from build123d import *

# Parameters (mm, degrees)
SKETCH1_W           = 25
SKETCH1_H           = 50
SKETCH1_R           = 3.375
BOSS_EXTRUDE1_DEPTH = 3
SKETCH2_W           = 50
SKETCH2_H           = 3
BOSS_EXTRUDE2_DEPTH = 8
SKETCH3_W           = 8
SKETCH3_H           = 50
BOSS_EXTRUDE3_DEPTH = 42
SKETCH4_R           = 2.65
CUT_EXTRUDE1_DEPTH  = 3.3
SKETCH5_R           = 5.802370205
CUT_EXTRUDE2_DEPTH  = 9
FILLET2_R           = 1
SKETCH6_R           = 12.7
BOSS_EXTRUDE4_DEPTH = 2
FILLET4_R           = 1
SKETCH8_R           = 1.589780168
SKETCH8_R_2         = 1.777428262
CUT_EXTRUDE3_DEPTH  = 10
SKETCH9_W           = 8
SKETCH9_H           = 42
CUT_EXTRUDE4_DEPTH  = 68.79439129
SKETCH10_W          = 33.517939775
SKETCH10_H          = 6.212330843
CUT_EXTRUDE5_DEPTH  = 55


with BuildPart() as part:
    # Sketch1 → Boss-Extrude1 (new body)
    with BuildSketch(Plane(origin=(0, 0, 0), x_dir=(1, 0, 0), z_dir=(0, 1, 0))):
        with Locations((2.276951673, 11.384758364)):
            Rectangle(SKETCH1_W, SKETCH1_H)
        with Locations(Location((1.276951673, 11.384758364, 0), (0, 0, 270))):
            Circle(SKETCH1_R, mode=Mode.SUBTRACT)
    extrude(amount=BOSS_EXTRUDE1_DEPTH)

    # Sketch2 → Boss-Extrude2 (add)
    with BuildSketch(Plane.ZY.offset(10.223048327)):
        with Locations((-11.384758364, 1.5)):
            Rectangle(SKETCH2_W, SKETCH2_H)
    extrude(amount=BOSS_EXTRUDE2_DEPTH)

    # Sketch3 → Boss-Extrude3 (add)
    with BuildSketch(Plane.XZ):
        with Locations((-14.223048327, -11.384758364)):
            Rectangle(SKETCH3_W, SKETCH3_H)
    extrude(amount=BOSS_EXTRUDE3_DEPTH)

    # Sketch4 → Cut-Extrude1 (cut)
    with BuildSketch(Plane(origin=(0, 3, 0), x_dir=(1, 0, 0), z_dir=(0, 1, 0))):
        with Locations(Location((-14.223048327, 32.384758364, 0), (0, 0, 270))):
            Circle(SKETCH4_R)
        with Locations(Location((-14.223048327, -9.615241636, 0), (0, 0, 270))):
            Circle(SKETCH4_R)
    cut_extrude1 = extrude(amount=-CUT_EXTRUDE1_DEPTH, mode=Mode.SUBTRACT)

    # Mirror1: Cut-Extrude1 across plane
    add(cut_extrude1.mirror(Plane.ZX.offset(-19.5)), mode=Mode.SUBTRACT)

    # Sketch5 → Cut-Extrude2 (cut)
    with BuildSketch(Plane.ZY.offset(18.223048327)):
        with Locations((-11.836279124, -21)):
            Circle(SKETCH5_R)
    extrude(amount=-CUT_EXTRUDE2_DEPTH, mode=Mode.SUBTRACT)

    # Fillet2
    fillet2_edges = [part.edges().sort_by_distance(p)[0] for p in [
        (-10.223048327, -21, -17.638649329),
    ]]
    fillet(fillet2_edges, radius=FILLET2_R)

    # Mirror2: Cut-Extrude1 across plane
    add(cut_extrude1.mirror(Plane.ZY.offset(1.723048327)), mode=Mode.SUBTRACT)

    # Sketch6 → Boss-Extrude4 (add)
    with BuildSketch(Plane(origin=(0, 3, 0), x_dir=(1, 0, 0), z_dir=(0, 1, 0))):
        with BuildLine():
            Line((14.776951673, 5.567542535), (14.776951673, 17.201974193))
            ThreePointArc((14.776951673, 17.201974193), (-13.423048327, 11.384758364), (14.776951673, 5.567542535))
        make_face()
        with Locations(Location((1.276951673, 11.384758364, 0), (0, 0, 270))):
            Circle(SKETCH6_R, mode=Mode.SUBTRACT)
    extrude(amount=BOSS_EXTRUDE4_DEPTH)

    # Fillet4
    # the kernel refuses this fillet: 1 mm, written as the material it takes off along each edge
    with BuildSketch(Plane(origin=(14.776951673, 5, -3.067542535), x_dir=(0, -1, 0), z_dir=(0, 0, -1))) as fillet4_piece_1:
        with BuildLine():
            CenterArc((FILLET4_R, FILLET4_R), FILLET4_R, 180, 90)
            Line((0, FILLET4_R), (0, 0))
            Line((0, 0), (FILLET4_R, 0))
        make_face()
    extrude(amount=16.634431658, mode=Mode.SUBTRACT)

    # Sketch8 → Cut-Extrude3 (cut)
    with BuildSketch(Plane(origin=(0, 3, 0), x_dir=(1, 0, 0), z_dir=(0, 1, 0))):
        with Locations(Location((1.276951673, 19.884758364, 0), (0, 0, 270))):
            Circle(SKETCH8_R)
        with Locations(Location((1.276951673, 2.884758364, 0), (0, 0, 270))):
            Circle(SKETCH8_R_2)
    extrude(amount=-CUT_EXTRUDE3_DEPTH, mode=Mode.SUBTRACT)

    # Sketch9 → Cut-Extrude4 (cut, through all)
    with BuildSketch(Plane.XY.offset(13.615241636)):
        with Locations((-14.223048327, -21)):
            Rectangle(SKETCH9_W, SKETCH9_H)
    extrude(amount=-CUT_EXTRUDE4_DEPTH, mode=Mode.SUBTRACT)

    # Sketch10 → Cut-Extrude5 (cut)
    with BuildSketch(Plane.XY.offset(13.615241636)):
        with Locations((-1.464078439, 6.106165422)):
            Rectangle(SKETCH10_W, SKETCH10_H)
    extrude(amount=-CUT_EXTRUDE5_DEPTH, mode=Mode.SUBTRACT)


solid = part.part
Source: CAD feature listing. Evaluate the final solid. Frame: model axes, mm. Coordinates: 2 decimals unless noted, no trailing zeros. Loops run counter-clockwise (first coordinate to the right, second up) from the corner with the lowest first, then second, coordinate; pieces in that order, holes last. Notation, with made-up numbers: (-38, 34) - (6, 34) arc R11 cw to (6, 54) - close; hole circle Ø3 at (-20.75, 32). An arc over 180 degrees is marked (long way). One line per item, written item: value. Start each with the question number.
1. Contact query for a flat-ended pin moving along its axis: P1, Ø6, axis at x = -14.22, z = -32.38, coming from the +Y side. Output: stop coordinate, or through.
2. Ray query, L1, parallel to Z at x = 9.5, y = 0.7; L2, parallel to Z at x = -15, y = 2.8; L3, parallel to Z at x = 0, y = 0.85. Return the intervals inside material, ascending.
3. Section C-C (y = 1.4). Return the cut outline in (x, z) (3 decimals).
4. Section B-B (x = 2). Return the cut outline in (y, z).
5. Section D-D (z = -9.5). Return the cut outline in (x, y), and give its area (3 significant figures).
6. Section A-A (z = -2). Return the cut outline in (x, y), and give its area (3 significant figures).
7. Mould query, pull axis Z, two halves, no side actions, for faces 1 (the flat face through (14.777, 1, -11)), 2 (the flat face through (-2, 2, 13.615)), 3 (the cylindrical face through (-11.596, 1.521, 9.27)). Classes: pulls with the +Z half, pulls with the -Z half, needs draft (parallel to the pull), parting line crosses it, or undercut.
Verdict:
1. P1: stops at y = 3
2. L1: z = -36.38 to -34.71, -30.06 to 7.29, 11.94 to 13.62
2. L2: z = -36.38 to -34.92, -29.85 to 7.08, 12.15 to 13.62
2. L3: z = -36.38 to -20.83, -18.94 to -14.51, -8.26 to -4.12, -1.65 to 13.62
3. outline: (-18.223, -36.385) - (14.777, -36.385) - (14.777, 13.615) - (-18.223, 13.615) - close; hole circle Ø5.3 at (-14.223, -32.385); hole circle Ø5.3 at (-14.223, 9.615); hole circle Ø6.75 at (1.277, -11.385); hole circle Ø3.555 at (1.277, -2.885); hole circle Ø3.18 at (1.277, -19.885); hole circle Ø5.3 at (10.777, -32.385); hole circle Ø5.3 at (10.777, 9.615)
4. outline: (0, -36.38) - (3, -36.38) - (3, -21.3) - (0, -21.3) - close; (0, -18.47) - (3, -18.47) - (3, -14.68) - (0, -14.68) - close; (0, -8.09) - (3, -8.09) - (3, -4.51) - (0, -4.51) - close; (0, -1.26) - (3, -1.26) - (3, 13.62) - (0, 13.62) - close
5. outline: (-18.22, 0) - (-1.52, 0) - (-1.52, 3) - (-18.22, 3) - close; (4.08, 0) - (14.78, 0) - (14.78, 3) - (4.08, 3) - close
5. area: 82.2 mm2
6. outline: (-18.22, 0) - (-0.26, 0) - (-0.26, 3) - (-18.22, 3) - close; (2.82, 0) - (14.78, 0) - (14.78, 3) - (2.82, 3) - close
6. area: 89.8 mm2
7. face 1: needs draft
7. face 2: pulls with the +Z half
7. face 3: undercut
